Autodesk Inventor part; units mm, degrees
ref_plane "YZ Plane" through (0, 0, 0) normal (1, 0, 0) x (0, 1, 0)
ref_plane "XZ Plane" through (0, 0, 0) normal (0, 1, 0) x (-1, 0, 0)
ref_plane "XY Plane" through (0, 0, 0) normal (0, 0, 1) x (1, 0, 0)
sketch "Эскиз1" plane through (0, 0, 0) normal (0, 0, 1) x (1, 0, 0)
  line L0 (-14.0097, -7.3348) -> (-16.3175, -6.3736)
  line L1 (-16.3175, -6.3736) -> (-14.0097, -7.3348)
  line L2 (17.7899, 2.7423) -> (-9.8124, 2.7423)
  line L3 (-14.0097, -7.3348) -> (-9.8124, 2.7423)
  line L4 (-9.8124, 2.7423) -> (17.7899, 2.7423)
  line L5 (-16.3175, -6.3736) -> (-6.7051, 16.7046)
  line L6 (-16.3175, -6.3736) -> (-6.7051, 16.7046)
  line L7 (-14.0257, -14.2577) -> (-10.5192, -14.2577)
  line L8 (-14.0257, -14.2577) -> (-10.5192, -14.2577)
  line L9 (-10.5192, -14.2577) -> (-10.5192, -12.2577)
  line L10 (-10.5192, -14.2577) -> (-10.5192, -12.2577)
  line L11 (-10.5192, -12.2577) -> (-12.5192, -12.2577)
  line L12 (-10.5192, -12.2577) -> (-12.5192, -12.2577)
  line L13 (-12.5192, -12.2577) -> (-12.5192, -10.2577)
  line L14 (-12.5192, -12.2577) -> (-12.5192, -10.2577)
  line L15 (-12.5192, -10.2577) -> (-9.4474, -10.2577)
  line L16 (-12.5192, -10.2577) -> (-9.4474, -10.2577)
  line L17 (-9.4474, -10.2577) -> (-6.5, 0.7423)
  line L18 (-9.4474, -10.2577) -> (-6.5, 0.7423)
  line L19 (-6.5, 0.7423) -> (6.5, 0.7423)
  line L20 (-6.5, 0.7423) -> (6.5, 0.7423)
  line L21 (9.4474, -10.2577) -> (12.5192, -10.2577)
  line L22 (6.5, 0.7423) -> (9.4474, -10.2577)
  line L23 (9.4474, -10.2577) -> (12.5192, -10.2577)
  line L24 (12.5192, -10.2577) -> (12.5192, -12.2577)
  line L25 (12.5192, -10.2577) -> (12.5192, -12.2577)
  line L26 (10.5192, -12.2577) -> (10.5192, -14.2577)
  line L27 (12.5192, -12.2577) -> (10.5192, -12.2577)
  line L28 (10.5192, -12.2577) -> (10.5192, -14.2577)
  line L29 (10.5192, -14.2577) -> (14.0257, -14.2577)
  arc A0 (17.7899, 2.7423) -> (-6.7051, 16.7046) centre (0, 0) ccw
  arc A1 (17.7899, 2.7423) -> (-6.7051, 16.7046) centre (0, 0) ccw
  arc A2 (17.5551, 2.9423) -> (-6.5528, 16.5499) centre (0, 0) ccw
  line L30 (17.5551, 2.9423) -> (-9.9457, 2.9423)
  line L31 (-14.1174, -7.0733) -> (-9.9457, 2.9423)
  line L32 (-16.056, -6.2659) -> (-6.5528, 16.5499)
  line L33 (-14.1174, -7.0733) -> (-16.056, -6.2659)
  arc A3 (-14.0257, -14.2577) -> (14.0257, -14.2577) centre (0, 0) ccw
  line L34 (13.5283, -14.4577) -> (10.3192, -14.4577)
  line L35 (10.3192, -12.0577) -> (10.3192, -14.4577)
  line L36 (12.3192, -12.0577) -> (10.3192, -12.0577)
  line L37 (12.3192, -10.4577) -> (12.3192, -12.0577)
  line L38 (9.294, -10.4577) -> (12.3192, -10.4577)
  line L39 (6.3465, 0.5423) -> (9.294, -10.4577)
  line L40 (-6.3465, 0.5423) -> (6.3465, 0.5423)
  line L41 (-9.294, -10.4577) -> (-6.3465, 0.5423)
  line L42 (-12.3192, -10.4577) -> (-9.294, -10.4577)
  line L43 (-12.3192, -12.0577) -> (-12.3192, -10.4577)
  line L44 (-10.3192, -12.0577) -> (-12.3192, -12.0577)
  line L45 (-10.3192, -14.4577) -> (-10.3192, -12.0577)
  line L46 (-14.0257, -14.4577) -> (-10.3192, -14.4577)
  line L47 (10.3192, -14.4577) -> (13.8194, -14.4577)
  point P0 (-13.8194, -14.4577)
  dimension "d9" = 0.2
  dimension "d10" = 0.2
  dimension "d11" = 0.2
  dimension "d12" = 0.2
  dimension "d13" = 0.2
  dimension "d15" = 0.2
  dimension "d16" = 0.2
  dimension "d17" = 0.2
  dimension "d18" = 0.2
  dimension "d19" = 0.2
  dimension "d20" = 0.2
  dimension "d21" = 0.2
  dimension "d22" = 0.2
  dimension "d23" = 0.2
  dimension "d24" = 0.2
  dimension "d25" = 0.2
  dimension "d26" = 0.2
  dimension "d27" = 3.5064
  dimension "d28" = 2
  dimension "d29" = 2
  dimension "d30" = 2
  dimension "d31" = 3.0718
  dimension "d32" = 11
  dimension "d33" = 13
  dimension "d34" = 11
  dimension "d35" = 3.0718
  dimension "d36" = 2
  dimension "d37" = 2
  dimension "d38" = 2
  dimension "d39" = 3.5064
  dimension "d40" = 20
  dimension "d41" = 2
  dimension "d42" = 0.2
extrude "Выдавливание1" add sketch "Эскиз1" along normal blind 3 contours L46 L45 L44 L43 L42 L41 L40 L39 L38 L37 L36 L35 L34 L47 A3 | L30 L31 L33 L32 A2
sketch "Эскиз3" plane through (0, 0, 3) normal (0, 0, 1) x (1, 0, 0)
  arc A0 (-19.1284, -5.8399) -> (-9.3269, 17.692) centre (0, 0) ccw
  arc A1 (-14.0257, -14.2577) -> (14.0257, -14.2577) centre (0, 0) ccw
  line L0 (-19.1284, -5.8399) -> (-9.3269, 17.692)
  line L1 (-6.5528, 16.5499) -> (-16.056, -6.2659)
  dimension "d43" = 3
extrude "Выдавливание3" add sketch "Эскиз3" along normal blind 2
chamfer "Фаска2" distance 0.5 angle 70 5 edges at (3.8047, 2.9423, 0) (8.7496, 15.5011, 0) (-11.3044, 5.142, 0) (-15.0867, -6.6696, 0) (-12.0316, -2.0655, 0) measured on face at (8.027, 4.2106, 0)
chamfer "Фаска3" distance 0.5 angle 70 12 edges at (7.8203, -4.9577, 0) (10.8066, -10.4577, 0) (12.3192, -11.2577, 0) (11.3192, -12.0577, 0) (10.3192, -13.2577, 0) (11.9238, -14.4577, 0) (-12.0693, -14.4577, 0) (-10.3192, -13.2577, 0) (-11.3192, -12.0577, 0) (-10.8066, -10.4577, 0) (-7.8203, -4.9577, 0) (0, 0.5423, 0) measured on face at (-1.9545, -6.8341, 0) measured on face at (1.7704, -6.791, 0) measured on face at (2.1155, -6.791, 0)
properties part number "cap2"
Could you check a few things on this model? Use its own coordinates, in mm. A direction names the side the tool comes from. Round coordinates to 2 decimals unless told otherwise and drop trailing zeros. Order: outer loops, then holes, each group sorted by start corner. A loop starts at its lowest first (then second) coordinate and runs counter-clockwise, first axis right, second up. Notation, with made-up numbers: (76, 71) -> (96, 71) arc R18 cw to (96, 88) -> close; hole circle Ø5 at (42.5, 41). An arc over 180 degrees is marked (long way). One line per question, with ' | ' between items.
Q1. Which directions (+Z, -Z, +X, -X, +Y, -Y) give clear straight access to the entire face, cutting with the end or side of a thin tool? Please do faces 4 (the face through (-11.37, 4.98, 2.18)), 5 (the face through (8.556, 15.609, 2.175)), 6 (the face through (7.61, -5.127, 0.696)), 7 (the face through (-10.319, -13, 2)).
Computed values:
face 4: -Z, -X, +Y | face 5: -Z, +Y | face 6: -Z, +X | face 7: -Z, -X
Q2. If we section it at A-A on z = 2.4: Write out the boundary of the cut face in (x, y), plus the area to 3 significant figures.
Computed values:
outline: (-16.06, -6.27) -> (-14.12, -7.07) -> (-9.95, 2.94) -> (17.56, 2.94) arc R17.8 ccw to (-6.55, 16.55) -> close; (-13.82, -14.46) arc R20 ccw to (13.82, -14.46) -> (10.32, -14.46) -> (10.32, -12.06) -> (12.32, -12.06) -> (12.32, -10.46) -> (9.29, -10.46) -> (6.35, 0.54) -> (-6.35, 0.54) -> (-9.29, -10.46) -> (-12.32, -10.46) -> (-12.32, -12.06) -> (-10.32, -12.06) -> (-10.32, -14.46) -> close | area: 718 mm²
Q3. If we section it at C-C on x = -7.5: Write out the boundary of the cut face in (y, z), plus the area to 3 significant figures.
Computed values:
outline: (-18.54, 0) -> (-5.69, 0) -> (-3.76, 1.37) -> (-3.76, 3) -> (2.94, 3) -> (2.94, 1.37) -> (3.44, 0) -> (12.98, 0) -> (14.28, 1.37) -> (14.28, 3) -> (18.54, 3) -> (18.54, 5) -> (-18.54, 5) -> close | area: 150 mm²
Q4. If we section it at D-D on y = -13: Write out the boundary of the cut face in (x, z), plus the area to 3 significant figures.
Computed values:
outline: (-15.2, 3) -> (-10.32, 3) -> (-10.32, 1.37) -> (-9.82, 0) -> (9.82, 0) -> (10.32, 1.37) -> (10.32, 3) -> (15.2, 3) -> (15.2, 5) -> (-15.2, 5) -> close | area: 122 mm²
Q5. If we section it at B-B on y = -0.5: Write out the boundary of the cut face in (x, z), plus the area to 3 significant figures.
Computed values:
outline: (-16.9, 3) -> (-13.65, 3) -> (-13.65, 1.37) -> (-13.11, 0) -> (-11.92, 0) -> (-11.38, 1.37) -> (-11.38, 3) -> (-6.63, 3) -> (-6.63, 1.37) -> (-6.11, 0) -> (6.11, 0) -> (6.63, 1.37) -> (6.63, 3) -> (19.99, 3) -> (19.99, 5) -> (-16.9, 5) -> close | area: 119 mm²
Q6. If I drill on line 1 (Y direction, x = -10.5, z = 1.8); line 2 (Z direction, x = 14, y = 10.5); line 3 (X direction, y = 0.5, z = 2.05), over which ranges is the centre line in solid material (lowest first)? Write a range as from..to.
Computed values:
line 1: -17.02..-14.46, -12.06..-10.46, 1.61..7.07 | line 2: 0.55..5 | line 3: -13.24..-10.96, -6.36..6.36
Q7. We'd pull the mould along Y, two halves only. Please class faces 1 (the face through (0, -20, 2)), 2 (the face through (-14.296, 5.761, 3.986)), 3 (the face through (11, -10.458, 2)): released by +Y, released by -Y, zero draft, split by the parting line, or undercut.
Computed values:
face 1: released by -Y | face 2: released by +Y | face 3: undercut
Q8. I'm going to push flat-ended pins straight in: pin 1 (1.3 mm diameter, centred on y = -11, z = 2, fed in from +X); pin 2 (0.5 mm diameter, centred on x = -11, z = 2.5, fed in from -Y); pin 3 (0.8 mm diameter, centred on y = -13.5, z = 2.5, fed in from +X). Where does each tip first touch, or does it pass through?
Computed values:
pin 1: x = 12.32 | pin 2: y = -16.87 | pin 3: x = 10.32
